Source: CAD feature listing. Evaluate the final solid. Frame: model axes, mm. Round coordinates to 2 decimals unless told otherwise and drop trailing zeros. Loops run counter-clockwise (first coordinate to the right, second up) from the corner with the lowest first, then second, coordinate; pieces in that order, holes last. Notation, with made-up numbers: M 44.25,19 L 52.25,19 A19 cw 52.25,36 Z; hole C 18,20 d2. An arc over 180 degrees is marked long. One line per item, written item: value.
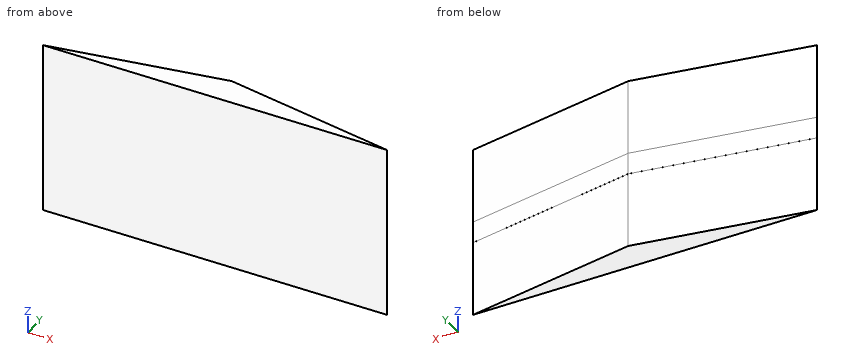
from build123d import *

# Parameters (mm, degrees)
EXTRUDE_1_DEPTH = 400
SKETCH_2_W      = 406.078810085
SKETCH_2_H      = 50
EXTRUDE_2_DEPTH = 0.1


with BuildPart() as part:
    # Эскиз1 → Бобышка-Вытянуть1 (new body)
    with BuildSketch(Plane.XY):
        Polygon((-400, 0), (400, 0), (0, 70), align=None)
    extrude(amount=EXTRUDE_1_DEPTH)

    # Эскиз2 → Бобышка-Вытянуть2 (add)
    with BuildSketch(Plane(origin=(11.88599151, 67.919951486, 0), x_dir=(0.9850304671557042, -0.17238033175224823, 0), z_dir=(0.17238033175224823, 0.9850304671557042, 0))):
        with Locations((190.972781819, -200)):
            Rectangle(SKETCH_2_W, SKETCH_2_H)
    extrude_2 = extrude(amount=EXTRUDE_2_DEPTH)

    # Зеркальное отражение1: Бобышка-Вытянуть2 across plane
    add(extrude_2.mirror(Plane(origin=(0, 0, 0), x_dir=(0, 0, 1), z_dir=(1, 0, 0))))


solid = part.part
1. Section query A-A (y = 29). Return the cut outline in (x, z), and give its area (3 significant figures).
Report:
outline: M -234.87,175 L -234.29,175 L -234.29,0 L 234.29,0 L 234.29,175 L 234.87,175 L 234.87,225 L 234.29,225 L 234.29,400 L -234.29,400 L -234.29,225 L -234.87,225 Z
area: 187,000 mm2
2. Pin query (flat end, axial travel): pin 1 (2 mm diameter, centred on x = -169, z = 259.5, fed in from +Y). Return the tip coordinate at first contact, or that it passes through.
Report:
pin 1: stops at y = 40.6
3. Section query C-C (z = 126). Return the cut outline in (x, y), and give its area (3 significant figures).
Report:
outline: M -400,0 L 400,0 L 0,70 Z
area: 28,000 mm2
4. Ray query, line 1 (Y direction, x = 0, z = 302); line 2 (Z direction, x = -226, y = 30.5); line 3 (Y direction, x = 170.5, z = 208). Return the intervals inside material, ascending. Write a range as [from, to].
Report:
line 1: y = [0, 70]
line 2: z = [175, 225]
line 3: y = [0, 40.26]
5. Section query D-D (x = 214). Return the cut outline in (y, z).
Report:
outline: M 0,0 L 32.55,0 L 32.55,175 L 32.65,175 L 32.65,225 L 32.55,225 L 32.55,400 L 0,400 Z
6. Section query B-B (x = -83). Return the cut outline in (y, z) (3 decimals), and give its area (3 significant figures).
Report:
outline: M 0,0 L 55.475,0 L 55.475,175 L 55.577,175 L 55.577,225 L 55.475,225 L 55.475,400 L 0,400 Z
area: 22,200 mm2
